from build123d import *

# Parameters (mm, degrees)
CROQUIS1_R              = 2.5
SALIENTE_EXTRUIR1_DEPTH = 12
REDONDEO1_R             = 10


with BuildPart() as part:
    # Croquis1 → Saliente-Extruir1 (new body)
    with BuildSketch(Plane(origin=(0, 0, 0), x_dir=(0, 0, -1), z_dir=(1, 0, 0))):
        with BuildLine():
            Line((-15, -30), (15, -30))
            Line((15, -30), (135, 5))
            Line((135, 5), (140, 5))
            ThreePointArc((140, 5), (145, 0), (140, -5))
            Line((140, -5), (135, -5))
            Line((135, -5), (15, -40))
            Line((15, -40), (-15, -40))
            Line((-15, -40), (-135, -5))
            Line((-135, -5), (-140, -5))
            ThreePointArc((-140, -5), (-145, 0), (-140, 5))
            Line((-140, 5), (-135, 5))
            Line((-135, 5), (-15, -30))
        make_face()
        with Locations((-8, -35)):
            Circle(CROQUIS1_R, mode=Mode.SUBTRACT)
        with Locations((8, -35)):
            Circle(CROQUIS1_R, mode=Mode.SUBTRACT)
        with Locations((-140, 0)):
            Circle(CROQUIS1_R, mode=Mode.SUBTRACT)
        with Locations((140, 0)):
            Circle(CROQUIS1_R, mode=Mode.SUBTRACT)
    extrude(amount=SALIENTE_EXTRUIR1_DEPTH)

    # Redondeo1
    redondeo1_edges = [part.edges().sort_by_distance(p)[0] for p in [
        (6, -5, -135),
        (6, -40, -15),
        (6, -40, 15),
        (6, -5, 135),
        (6, 5, 135),
        (6, -30, 15),
        (6, -30, -15),
        (6, 5, -135),
    ]]
    fillet(redondeo1_edges, radius=REDONDEO1_R)


solid = part.part
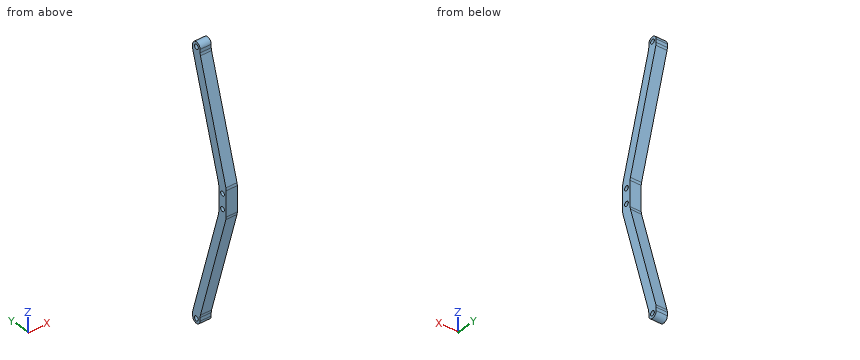
Verification items for the finished model (mm, model axes). Coordinates: 2 decimals unless noted, no trailing zeros. Order: outer loops, then holes, each group sorted by start corner. A loop starts at its lowest first (then second) coordinate and runs counter-clockwise, first axis right, second up. Notation, with made-up numbers: M 87.5,74.5 L 110.5,74.5 A34 cw 110.5,106.5 Z; hole C 34.5,-32.75 d1. An arc over 180 degrees is marked long. Return JSON: item names as keys, results as strings.
1) Cross-section at C-C, the plane y = -35. Record the boundary of the cut face in (x, z), and give its area (3 significant figures).
Answer list:
{"outline": "M 0,-32.14 L 12,-32.14 L 12,-10.5 L 0,-10.5 Z; M 0,-5.5 L 12,-5.5 L 12,5.5 L 0,5.5 Z; M 0,10.5 L 12,10.5 L 12,32.14 L 0,32.14 Z", "area": "651 mm2"}
2) Cross-section at B-B, the plane y = -21. Record the boundary of the cut face in (x, z), and give its area (3 significant figures).
Answer list:
{"outline": "M 0,-80.14 L 12,-80.14 L 12,-45.86 L 0,-45.86 Z; M 0,45.86 L 12,45.86 L 12,80.14 L 0,80.14 Z", "area": "823 mm2"}
3) Cross-section at A-A, the plane z = -8. Record the boundary of the cut face in (x, y), and give its area (3 significant figures).
Answer list:
{"outline": "M 0,-40 L 12,-40 L 12,-37.5 L 0,-37.5 Z; M 0,-32.5 L 12,-32.5 L 12,-30 L 0,-30 Z", "area": "60.0 mm2"}
4) Cross-section at D-D, the plane y = 0. Record the boundary of the cut face in (x, z), and give its area (3 significant figures).
Answer list:
{"outline": "M 0,-145 L 12,-145 L 12,-142.5 L 0,-142.5 Z; M 0,-137.5 L 12,-137.5 L 12,-117.86 L 0,-117.86 Z; M 0,117.86 L 12,117.86 L 12,137.5 L 0,137.5 Z; M 0,142.5 L 12,142.5 L 12,145 L 0,145 Z", "area": "531 mm2"}
5) Gauge pin test, flat ends, axial feed: pin 1 (3.5 mm diameter, centred on x = 9, z = 0, fed in from +Y); pin 2 (1.8 mm diameter, centred on x = 8.5, z = -138, fed in from -Y); pin 3 (1.5 mm diameter, centred on x = 3, z = -114.5, fed in from +Y). Record the tip position at first contact, or that the pin passes through.
Answer list:
{"pin 1": "y = -30", "pin 2": "y = -5", "pin 3": "y = -0.76"}
6) Thickness scan on L1, parallel to Y at x = 7, z = 8; L2, parallel to Y at x = 4.5, z = -140; L3, parallel to Y at x = 3.25, z = 11. Record the ranges inside material, lowest first. Write a range as [from, to].
Answer list:
{"L1": "[-40, -37.5], [-32.5, -30]", "L2": "[-5, -2.5], [2.5, 5]", "L3": "[-40, -30]"}
